Source: CAD feature listing. Evaluate the final solid. Frame: model axes, mm. A direction names the side the tool comes from. Coordinates: 2 decimals unless noted, no trailing zeros. Write each loop counter-clockwise with the first axis right and the second up, starting at its lowest first coordinate (ties: lowest second). Pieces come first, ordered by that corner, then holes. Notation, with made-up numbers: M 67.25,74.5 L 95.25,74.5 A32 ccw 95.25,104.5 Z; hole C 87.5,68.5 d11. An arc over 180 degrees is marked long. One line per item, written item: value. Start each with the question number.
Item 1: Cut plane A-A, the plane y = 0. Output: boundary loops of the cut face in (x, z).
Item 2: Mould query, pull axis X, two halves, no side actions, for faces 1 (the flat face through (-32, 28, 15)), 2 (the cylindrical face through (-11.923, -53.692, 0.182)), 3 (the conical face through (-8.698, -39.171, -13.125)). Classes: released by +X, released by -X, zero draft, split by the parting line, or undercut.
Item 3: Pin query (flat end, axial travel): P1, Ø2, axis at x = -40, z = 5.5, coming from the -Y side; P2, Ø2, axis at x = -15, y = -38, coming from the -Z side; P3, Ø1, axis at x = -19, z = 7, coming from the +Y side. Return the tip coordinate at first contact, or that it passes through.
Item 4: Cut plane C-C, the plane z = -5.75. Output: boundary loops of the cut face in (x, y).
Item 5: Set-up query: faces 4 (the flat face through (-32, 28, -15)), 5 (the cylindrical face through (9.43, -42.466, -1.288)). Return all of +Z, -Z, +X, -X, +Y, -Y with unobstructed straight access to the full face (end or side cutting, diameter ignored); none if empty.
Item 6: Ray query, L1, parallel to Y at x = 0, z = 10.75; L2, parallel to Y at x = 0, z = -2.55; L3, parallel to X at y = -1, z = 2.25. Return the intervals inside material, ascending. Write a range as from..to.
```python
from build123d import *

# Parameters (mm, degrees)
SKETCH1_R           = 55
SKETCH1_R_2         = 40
BOSS_EXTRUDE1_DEPTH = 15
CHAMFER1_SIZE       = 2
SKETCH2_W           = 7.914202957
SKETCH2_H           = 5.5


with BuildPart() as part:
    # Sketch1 → Boss-Extrude1 (new body, symmetric)
    with BuildSketch(Plane.XY):
        Circle(SKETCH1_R)
        Circle(SKETCH1_R_2, mode=Mode.SUBTRACT)
    extrude(amount=BOSS_EXTRUDE1_DEPTH, both=True)

    # Chamfer1
    chamfer1_edges = [part.edges().sort_by_distance(p)[0] for p in [
        (-55, 0, -15),
        (-55, 0, 15),
        (-40, 0, -15),
        (-40, 0, 15),
    ]]
    chamfer(chamfer1_edges, length=CHAMFER1_SIZE)

    # Sketch2 → Cut-Revolve1 (revolve, cut)
    with BuildSketch(Plane(origin=(0, 0, 0), x_dir=(1, 0, 0), z_dir=(0, 1, 0))):
        with Locations((-39.542898521, 1.25)):
            Rectangle(SKETCH2_W, SKETCH2_H)
    revolve(axis=Axis((0, 0, 0), (0, 0, -1)), mode=Mode.SUBTRACT)


solid = part.part
```
From the geometry:
1. outline: M -55,-13 L -53,-15 L -42,-15 L -40,-13 L -40,-4 L -43.5,-4 L -43.5,1.5 L -40,1.5 L -40,13 L -42,15 L -53,15 L -55,13 Z; M 40,-13 L 42,-15 L 53,-15 L 55,-13 L 55,13 L 53,15 L 42,15 L 40,13 L 40,1.5 L 43.5,1.5 L 43.5,-4 L 40,-4 Z
2. face 1: zero draft
2. face 2: split by the parting line
2. face 3: undercut
3. P1: stops at y = -38.78
3. P2: stops at z = -14.85
3. P3: stops at y = 51.8
4. outline: C 0,0 d110; hole C 0,0 d80
5. face 4: -Z, +X, -X, +Y, -Y
5. face 5: none
6. L1: y = -55..-40, 40..55
6. L2: y = -55..-43.5, 43.5..55
6. L3: x = -54.99..-39.99, 39.99..54.99
